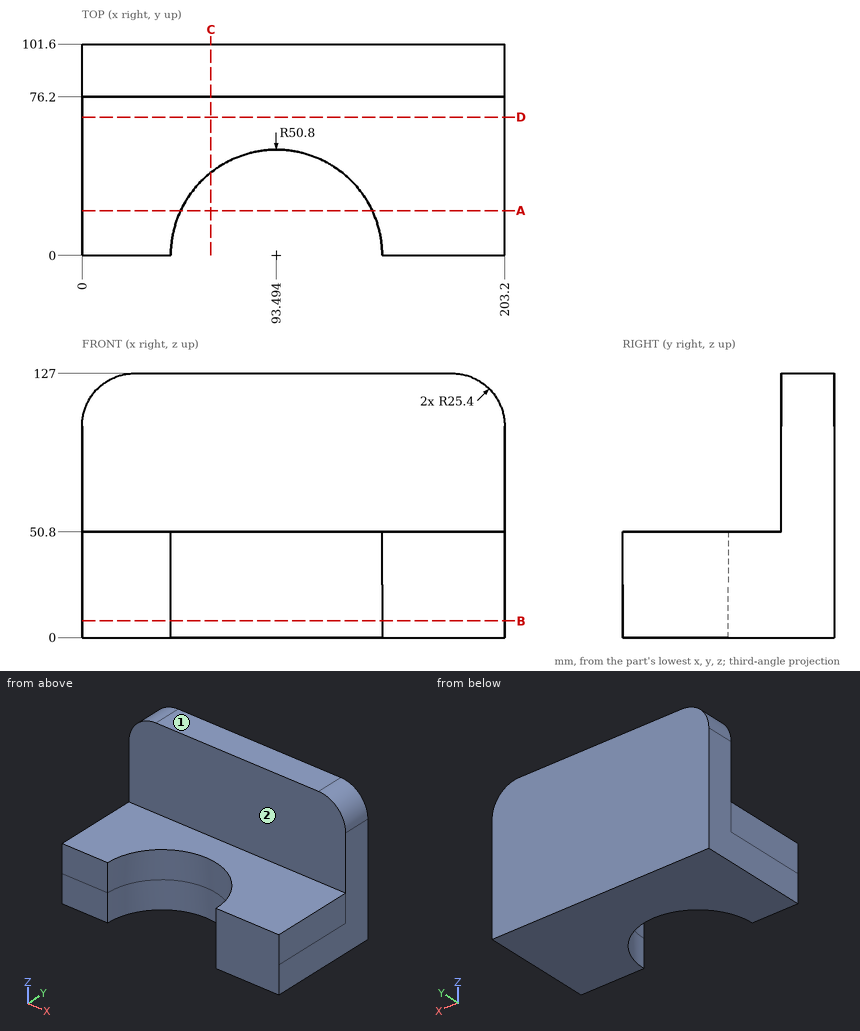
Geometry: see drawing. Coordinates: mm, zero at the bounding-box minimum. A direction names the side the tool comes from. Give positions to 0.01 mm unless a question says otherwise; leave off trailing zeros. Write each loop counter-clockwise with the first axis right and the second up, starting at its lowest first coordinate (ties: lowest second). Pieces come first, ordered by that corner, then holes. Notation, with made-up numbers: (20, 89.25) - (69, 89.25) arc R14 ccw to (69, 101.25) - close; hole circle Ø2 at (84, 27). An arc over 180 degrees is marked (long way). Return JSON: item names as keys, results as strings. Group by question number.
1) Section C-C on x = 62. Return the cut outline in (y, z), plus the area to 3 significant figures.
2) First-contact query: P1, Ø8, axis at x = 38.5, z = 110, coming from the -Y side; P2, Ø10, axis at x = 88.5, y = 62, coming from the +Z side. Flat tips, straight axial feed; report the tip coordinate or a pass-through.
3) Set-up query: the marked faces 1 and 2. Return all of +Z, -Z, +X, -X, +Y, -Y with unobstructed straight access to the full face (end or side cutting, diameter ignored); none if empty.
4) Section B-B on z = 8. Return the cut outline in (x, y).
5) Section A-A on y = 21.5. Return the cut outline in (x, z).
6) Section D-D on y = 66.5. Return the cut outline in (x, z), plus the area to 3 significant figures.
7) Line query: line 1 (Z direction, x = 17, y = 27.5); line 2 (Y direction, x = 110, z = 74.5); line 3 (Z direction, x = 178.5, y = 78.5). Output: solid intervals per line, ascending.
Filled in:
{
 "1": {"outline": "(39.86, 0) - (101.6, 0) - (101.6, 127) - (76.2, 127) - (76.2, 50.8) - (39.86, 50.8) - close", "area": "5,070 mm^2"},
 "2": {"P1": "stops at y = 76.2", "P2": "stops at z = 50.8"},
 "3": {"face 1": "+Z, +X, -X, +Y, -Y", "face 2": "+Z, +X, -X, -Y"},
 "4": {"outline": "(0, 0) - (42.69, 0) arc R50.8 cw to (144.29, 0) - (203.2, 0) - (203.2, 101.6) - (0, 101.6) - close"},
 "5": {"outline": "(0, 0) - (47.47, 0) - (47.47, 50.8) - (0, 50.8) - close; (139.52, 0) - (203.2, 0) - (203.2, 50.8) - (139.52, 50.8) - close"},
 "6": {"outline": "(0, 0) - (203.2, 0) - (203.2, 50.8) - (0, 50.8) - close", "area": "10,300 mm^2"},
 "7": {"line 1": "z = 0 to 50.8", "line 2": "y = 76.2 to 101.6", "line 3": "z = 0 to 126.99"}
}
